Design review of the part built by this model. Coordinates are the model's own, in mm. A direction names the side the tool comes from. Give positions to 0.01 mm unless a question says otherwise; leave off trailing zeros. Loops run counter-clockwise (first coordinate to the right, second up) from the corner with the lowest first, then second, coordinate; pieces in that order, holes last. Notation, with made-up numbers: (41.25, 49.25) -> (55.25, 49.25) arc R19 ccw to (55.25, 72.25) -> close; hole circle Ø1 at (27, 58.5). An arc over 180 degrees is marked (long way). Use a Markdown table: item, result. Add a question column.
1. Add section C-C (x = 18.5). Count the separate pieces of the cut face and the enclosed holes in it, and give its area (3 significant figures).
2. To check wall thickness, follow line 1 (Y direction, x = 6.5, z = 40); line 2 (Z direction, x = 11, y = 36.5). State the ranges of each line that lie inside material, in increasing order.
3. Add section A-A (x = 8). State the section outline as (y, z) points (3 decimals), and give its area (3 significant figures).
4. Draft analysis for pull direction Y (two halves, no side actions). For faces 1 (the cylindrical face through (16.097, 1.528, 1.449)), 2 (the conical face through (15.948, 38.523, 0.159)), 3 (the conical face through (12.935, 12.669, 0.159)), 4 (the flat face through (16, 1, 47.625)), state which applies: pulls with the +Y half, pulls with the -Y half, needs draft (parallel to the pull), parting line crosses it, or undercut.
5. For pin 1 Ø6 at (y, z) = (6, 13) entering from -X; pin 2 Ø16 at (x, z) = (23.5, 24) entering from +Y; pin 3 Ø5 at (x, y) = (9, 24) entering from +Z; pin 4 Ø8 at (x, y) = (14.5, 36.5) entering from +Z, all flat-tipped, find the tip position at first contact; note any pin that passes through.
6. For faces 5 (the flat face through (16, 27, 2.54)), 6 (the cylindrical face through (1.086, 1.288, 46.479)), list the 3-axis set-ups (+Z, -Z, +X, -X, +Y, -Y) from which the entire face can be reached by the end or side of a thin tool; tool diameter is ignored.
7. Add section D-D (x = 29.5). State the section outline as (y, z) points, and give its area (3 significant figures).
8. Add section B-B (y = 6). State the section outline as (x, z) points, and give its area (3 significant figures).
```python
from build123d import *

# Parameters (mm, degrees)
SKETCH1_W                                      = 31.75
SKETCH1_H                                      = 47.625
BOSS_EXTRUDE1_DEPTH                            = 2.54
SKETCH3_W                                      = 31.75
SKETCH3_H                                      = 45.085
BOSS_EXTRUDE2_DEPTH                            = 2.54
FILLET1_R                                      = 5.08
FILLET2_R                                      = 2.54
FILLET3_R                                      = 3.81
CSK_FOR_1_4_FLAT_HEAD_MACHINE_SCREW_2_COUNT    = 2
CSK_FOR_1_4_FLAT_HEAD_MACHINE_SCREW_2_PITCH    = 20.320445496
CSK_FOR_1_4_FLAT_HEAD_MACHINE_SCREW_3_AT_COUNT = 2
CSK_FOR_1_4_FLAT_HEAD_MACHINE_SCREW_3_AT_PITCH = 20.32


with BuildPart() as part:
    # Sketch1 → Boss-Extrude1 (new body)
    with BuildSketch(Plane.XY):
        with Locations((15.875, 23.8125)):
            Rectangle(SKETCH1_W, SKETCH1_H)
    extrude(amount=BOSS_EXTRUDE1_DEPTH)

    # Sketch3 → Boss-Extrude2 (add)
    with BuildSketch(Plane.XZ):
        with Locations((15.875, 25.0825)):
            Rectangle(SKETCH3_W, SKETCH3_H)
    extrude(amount=-BOSS_EXTRUDE2_DEPTH)

    # Fillet1
    fillet1_edges = [part.edges().sort_by_distance(p)[0] for p in [
        (15.875, 0, 0),
    ]]
    fillet(fillet1_edges, radius=FILLET1_R)

    # Fillet2
    fillet2_edges = [part.edges().sort_by_distance(p)[0] for p in [
        (15.875, 2.54, 2.54),
    ]]
    fillet(fillet2_edges, radius=FILLET2_R)

    # Fillet3
    fillet3_edges = [part.edges().sort_by_distance(p)[0] for p in [
        (0, 1.27, 47.625),
        (31.75, 1.27, 47.625),
        (0, 47.625, 1.27),
        (31.75, 47.625, 1.27),
    ]]
    fillet(fillet3_edges, radius=FILLET3_R)

    # Sketch5 → CSK for 1_4 Flat Head Machine Screw _100 (revolve, cut)
    with BuildSketch(Plane(origin=(16.106267099, 34.925, 2.54), x_dir=(0, -1, 0), z_dir=(1, 0, 0))):
        Polygon((0, 0), (0, 2.54), (3.3782, 2.54), (3.3782, 2.568232241), (6.4389, 0), align=None)
    csk_for_1_4_flat_head_machine_screw_100 = revolve(axis=Axis((16.106267099, 34.925, 8.89), (0, 0, -1)), mode=Mode.SUBTRACT)

    # CSK for 1_4 Flat Head Machine Screw  2: CSK for 1_4 Flat Head Machine Screw _100 ×2
    with Locations(*[Vector(-0.006621675847692915, -0.9999780764641634, 0) * (i * CSK_FOR_1_4_FLAT_HEAD_MACHINE_SCREW_2_PITCH) for i in range(1, CSK_FOR_1_4_FLAT_HEAD_MACHINE_SCREW_2_COUNT)]):
        add(csk_for_1_4_flat_head_machine_screw_100, mode=Mode.SUBTRACT)

    # Sketch7 → CSK for 1_4 Flat Head Machine Screw  3 (revolve, cut)
    with BuildSketch(Plane(origin=(15.875, 2.54, 34.925), x_dir=(0, 0, 1), z_dir=(1, 0, 0))):
        Polygon((0, 0), (0, 2.54), (3.3782, 2.54), (3.3782, 2.568232241), (6.4389, 0), align=None)
    csk_for_1_4_flat_head_machine_screw_3 = revolve(axis=Axis((15.875, 8.89, 34.925), (0, -1, 0)), mode=Mode.SUBTRACT)

    # CSK for 1_4 Flat Head Machine Screw 3 at: CSK for 1_4 Flat Head Machine Screw  3 ×2
    with Locations(*[(0, 0, -i * CSK_FOR_1_4_FLAT_HEAD_MACHINE_SCREW_3_AT_PITCH) for i in range(1, CSK_FOR_1_4_FLAT_HEAD_MACHINE_SCREW_3_AT_COUNT)]):
        add(csk_for_1_4_flat_head_machine_screw_3, mode=Mode.SUBTRACT)


solid = part.part
```
Taken from the geometry:
| question | item | result |
|---|---|---|
| 1 | separate pieces | 5 |
| 1 | enclosed holes | 0 |
| 1 | area | 146 mm^2 |
| 2 | line 1 | y = 0 to 2.54 |
| 2 | line 2 | z = 0 to 1.62 |
| 3 | outline | (0, 5.08) arc R5.08 ccw to (5.08, 0) -> (47.625, 0) -> (47.625, 2.54) -> (5.08, 2.54) arc R2.54 cw to (2.54, 5.08) -> (2.54, 47.625) -> (0, 47.625) -> close |
| 3 | area | 231 mm^2 |
| 4 | face 1 | pulls with the -Y half |
| 4 | face 2 | undercut |
| 4 | face 3 | undercut |
| 4 | face 4 | needs draft |
| 5 | pin 1 | passes through |
| 5 | pin 2 | stops at y = 2.54 |
| 5 | pin 3 | stops at z = 2.54 |
| 5 | pin 4 | stops at z = 2.38 |
| 6 | face 5 | +Z, +X, -X, +Y |
| 6 | face 6 | +Z, -X, +Y, -Y |
| 7 | outline | (0, 5.08) arc R5.08 ccw to (5.08, 0) -> (47.29, 0) -> (47.29, 2.54) -> (5.08, 2.54) arc R2.54 cw to (2.54, 5.08) -> (2.54, 47.29) -> (0, 47.29) -> close |
| 7 | area | 230 mm^2 |
| 8 | outline | (0, 0) -> (31.75, 0) -> (31.75, 2.54) -> (0, 2.54) -> close |
| 8 | area | 80.6 mm^2 |
